For this review, take the finished solid that the model builds, in its own axes (mm). Give positions to 0.01 mm unless a question says otherwise; leave off trailing zeros. Return JSON: item names as keys, results as strings.
Autodesk Inventor part; units mm, degrees
ref_plane "YZ Plane" through (0, 0, 0) normal (1, 0, 0) x (0, 1, 0)
ref_plane "XZ Plane" through (0, 0, 0) normal (0, 1, 0) x (-1, 0, 0)
ref_plane "XY Plane" through (0, 0, 0) normal (0, 0, 1) x (1, 0, 0)
sketch "Sketch1" plane through (0, 0, 0) normal (0, 1, 0) x (-1, 0, 0)
  line L0 (3.9, -2.8393) -> (3.9, 2.8393)
  line L1 (2.8393, 3.9) -> (-2.8393, 3.9)
  line L2 (-2.8393, -3.9) -> (2.8393, -3.9)
  line L3 (8.5707, 3.2957) -> (10, 4.725)
  line L4 (8.5707, -3.2957) -> (10, -4.725)
  line L5 (8.4, 3.3664) -> (8.4, 6)
  line L6 (8.4, 6) -> (7.0607, 6)
  line L7 (10, 9) -> (10, 4.725)
  line L8 (10, -4.725) -> (10, -9)
  line L9 (3.9, 2.8393) -> (7.0607, 6)
  line L10 (3.2957, 8.5707) -> (4.725, 10)
  line L11 (3.3664, 8.4) -> (6, 8.4)
  line L12 (6, 8.4) -> (6, 7.0607)
  line L13 (2.8393, 3.9) -> (6, 7.0607)
  line L14 (8.4, -3.3664) -> (8.4, -6)
  line L15 (8.4, -6) -> (7.0607, -6)
  line L16 (3.9, -2.8393) -> (7.0607, -6)
  line L17 (3.2957, -8.5707) -> (4.725, -10)
  line L18 (3.3664, -8.4) -> (6, -8.4)
  line L19 (6, -8.4) -> (6, -7.0607)
  line L20 (2.8393, -3.9) -> (6, -7.0607)
  line L21 (-3.9, -2.8393) -> (-3.9, 2.8393)
  line L22 (-3.9, 2.8393) -> (-7.0607, 6)
  line L23 (-6, 8.4) -> (-6, 7.0607)
  line L24 (-2.8393, 3.9) -> (-6, 7.0607)
  line L25 (-3.9, -2.8393) -> (-7.0607, -6)
  line L26 (-2.8393, -3.9) -> (-6, -7.0607)
  line L27 (-6, -8.4) -> (-6, -7.0607)
  line L28 (-3.3664, -8.4) -> (-6, -8.4)
  line L29 (-3.2957, -8.5707) -> (-4.725, -10)
  line L30 (4.725, 10) -> (9, 10)
  line L31 (9, -10) -> (4.725, -10)
  circle A0 centre (0, 0) radius 2.1
  arc A1 (10, 9) -> (9, 10) centre (9, 9) ccw
  arc A2 (9, -10) -> (10, -9) centre (9, -9) ccw
  arc A3 (8.4, 3.3664) -> (8.5707, 3.2957) centre (8.5, 3.3664) ccw
  arc A4 (3.2957, 8.5707) -> (3.3664, 8.4) centre (3.3664, 8.5) ccw
  arc A5 (8.5707, -3.2957) -> (8.4, -3.3664) centre (8.5, -3.3664) ccw
  arc A6 (3.3664, -8.4) -> (3.2957, -8.5707) centre (3.3664, -8.5) ccw
  arc A7 (-3.2957, -8.5707) -> (-3.3664, -8.4) centre (-3.3664, -8.5) ccw
  line L32 (-23.9, -2.8393) -> (-23.9, 2.8393)
  line L33 (-22.8393, 3.9) -> (-17.1607, 3.9)
  line L34 (-17.1607, -3.9) -> (-22.8393, -3.9)
  line L35 (-28.5707, 3.2957) -> (-30, 4.725)
  line L36 (-28.5707, -3.2957) -> (-30, -4.725)
  line L37 (-28.4, 3.3664) -> (-28.4, 6)
  line L38 (-28.4, 6) -> (-27.0607, 6)
  line L39 (-30, 9) -> (-30, 4.725)
  line L40 (-30, -4.725) -> (-30, -9)
  line L41 (-23.9, 2.8393) -> (-27.0607, 6)
  line L42 (-23.2957, 8.5707) -> (-24.725, 10)
  line L43 (-23.3664, 8.4) -> (-26, 8.4)
  line L44 (-26, 8.4) -> (-26, 7.0607)
  line L45 (-22.8393, 3.9) -> (-26, 7.0607)
  line L46 (-23.9, 0) -> (-28.4, 0)
  line L47 (-23.9, -2.8393) -> (-27.0607, -6)
  line L48 (-28.4, -6) -> (-27.0607, -6)
  line L49 (-28.4, -3.3664) -> (-28.4, -6)
  line L50 (-22.8393, -3.9) -> (-26, -7.0607)
  line L51 (-26, -8.4) -> (-26, -7.0607)
  line L52 (-23.3664, -8.4) -> (-26, -8.4)
  line L53 (-23.2957, -8.5707) -> (-24.725, -10)
  line L54 (-16.1, -2.8393) -> (-12.9393, -6)
  line L55 (-17.1607, -3.9) -> (-14, -7.0607)
  line L56 (-16.6336, -8.4) -> (-14, -8.4)
  line L57 (-16.1, -2.8393) -> (-16.1, 2.8393)
  line L58 (-16.1, 2.8393) -> (-12.9393, 6)
  line L59 (-17.1607, 3.9) -> (-14, 7.0607)
  line L60 (-14, 8.4) -> (-14, 7.0607)
  line L61 (-14, -8.4) -> (-14, -7.0607)
  line L62 (-16.7043, -8.5707) -> (-15.275, -10)
  line L63 (-24.725, 10) -> (-29, 10)
  line L64 (-29, -10) -> (-24.725, -10)
  circle A8 centre (-20, 0) radius 2.1
  arc A9 (-29, 10) -> (-30, 9) centre (-29, 9) ccw
  arc A10 (-30, -9) -> (-29, -10) centre (-29, -9) ccw
  arc A11 (-28.5707, 3.2957) -> (-28.4, 3.3664) centre (-28.5, 3.3664) ccw
  arc A12 (-23.3664, 8.4) -> (-23.2957, 8.5707) centre (-23.3664, 8.5) ccw
  arc A13 (-28.4, -3.3664) -> (-28.5707, -3.2957) centre (-28.5, -3.3664) ccw
  arc A14 (-23.2957, -8.5707) -> (-23.3664, -8.4) centre (-23.3664, -8.5) ccw
  arc A15 (-16.6336, -8.4) -> (-16.7043, -8.5707) centre (-16.6336, -8.5) ccw
  arc A16 (-16.7043, 8.5707) -> (-16.6336, 8.4) centre (-16.6336, 8.5) ccw
  line L65 (-7.5, -8.4) -> (-7.5, -6.4393)
  line L66 (-7.0607, -6) -> (-7.5, -6.4393)
  line L67 (-12.5, -7.0607) -> (-12.5, -8.4)
  line L68 (-12.9393, -6) -> (-12.5, -6.4393)
  line L69 (-12.5, -6.4393) -> (-12.5, -7.0607)
  line L70 (-7.5, -8.4) -> (-12.5, -8.4)
  line L71 (-4.725, -10) -> (-15.275, -10)
  line L72 (-3.9, 2.8393) -> (-7.0607, 6)
  line L73 (-2.8393, 3.9) -> (-6, 7.0607)
  line L74 (-3.3664, 8.4) -> (-6, 8.4)
  line L75 (-6, 8.4) -> (-6, 7.0607)
  line L76 (-3.2957, 8.5707) -> (-4.725, 10)
  arc A17 (-3.3664, 8.4) -> (-3.2957, 8.5707) centre (-3.3664, 8.5) ccw
  line L77 (-16.1, 2.8393) -> (-12.9393, 6)
  line L78 (-17.1607, 3.9) -> (-14, 7.0607)
  line L79 (-16.6336, 8.4) -> (-14, 8.4)
  line L80 (-14, 8.4) -> (-14, 7.0607)
  line L81 (-16.7043, 8.5707) -> (-15.275, 10)
  arc A18 (-16.7043, 8.5707) -> (-16.6336, 8.4) centre (-16.6336, 8.5) ccw
  line L82 (-7.5, 8.4) -> (-7.5, 6.4393)
  line L83 (-7.0607, 6) -> (-7.5, 6.4393)
  line L84 (-12.5, 7.0607) -> (-12.5, 8.4)
  line L85 (-12.9393, 6) -> (-12.5, 6.4393)
  line L86 (-12.5, 6.4393) -> (-12.5, 7.0607)
  line L87 (-7.5, 8.4) -> (-12.5, 8.4)
  line L88 (-4.725, 10) -> (-15.275, 10)
extrude "Extrusion1" add sketch "Sketch1" along normal blind 620
properties part number "VSLOT20x40x620"
1. For pin 1 (10 mm diameter, centred on y = 487.5, z = 3, fed in from +X); pin 2 (1 mm diameter, centred on x = 16, y = 134.5, fed in from -Z) (3 decimals); pin 3 (6 mm diameter, centred on y = 398.5, z = -1, fed in from +X) (3 decimals); pin 4 (1.7 mm diameter, centred on x = 20, y = 402, fed in from -Z), all flat-tipped, find the tip position at first contact; note any pin that passes through.
Results found:
{"pin 1": "stops at x = 30", "pin 2": "stops at z = -9.775", "pin 3": "stops at x = 29.275", "pin 4": "stops at z = -3.9"}
2. Add section A-A, the plane y = 390. Count the separate pieces of the cut face and the enclosed holes in it, plus the area to 3 significant figures.
Results found:
{"separate pieces": "1", "enclosed holes": "3", "area": "281 mm²"}
3. To check wall thickness, follow probe 1 along X at (y, z) = (197.5, 8); probe 2 along Z at (x, y) = (0, 445); probe 3 along X at (y, z) = (462, 4.5) (3 decimals). State the ranges of each line that lie inside material, in increasing order.
Results found:
{"probe 1": "x = -10 to -6, 6 to 7.5, 12.5 to 14, 26 to 30", "probe 2": "z = -3.9 to -2.1, 2.1 to 3.9", "probe 3": "x = -9.775 to -8.4, -5.561 to -3.439, 3.439 to 5.561, 14.439 to 16.561, 23.439 to 25.561, 28.4 to 29.775"}
